from build123d import *

# Parameters (mm, degrees)
F0_R            = 75
F1_DEPTH        = 5
F2_W            = 78
F2_H            = 78
F2_W_2          = 76
F2_H_2          = 76
F2_W_3          = 56
F2_H_3          = 56
F2_W_4          = 54
F2_H_4          = 54
F3_DEPTH        = 1
F4_R            = 1
F5_DEPTH        = 5.001
F5_COPIES_COUNT = 3


# Not quite as in the source:
# - a pattern or mirror of a feature is missing from the dataset's text; its kind, count and spacing are read off the source's solid


with BuildPart() as f1:
    # F0 (on Top) → F1 (new body)
    with BuildSketch(Plane.XY):
        Circle(F0_R)
    extrude(amount=F1_DEPTH)

    # F2 (on face) → F3 (cut)
    with BuildSketch(Plane.XY.offset(5)):
        Rectangle(F2_W, F2_H)
        Rectangle(F2_W_2, F2_H_2, mode=Mode.SUBTRACT)
        Rectangle(F2_W_3, F2_H_3)
        Rectangle(F2_W_4, F2_H_4, mode=Mode.SUBTRACT)
    extrude(amount=-F3_DEPTH, mode=Mode.SUBTRACT)

    # F4 (on face) → F5 (cut, through all)
    with BuildSketch(Plane.XY.offset(5)):
        with Locations((0, 70)):
            Circle(F4_R)
        with Locations((3.663516937, 69.9040674328)):
            Circle(F4_R)
        with Locations((7.3169924287, 69.6165326758)):
            Circle(F4_R)
    f5 = extrude(amount=-F5_DEPTH, mode=Mode.SUBTRACT)

    # F5_copies: F5 ×3 about axis
    f5_copies_axis = Axis((0, 0, 0), (0, 0, 1))
    for i in range(1, F5_COPIES_COUNT):
        add(f5.rotate(f5_copies_axis, i * 360 / F5_COPIES_COUNT), mode=Mode.SUBTRACT)


solid = f1.part
Input: part model. Units: mm. Frame: model coordinates. Give positions to 0.01 mm unless a question says otherwise; leave off trailing zeros. Order: outer loops, then holes, each group sorted by start corner. A loop starts at its lowest first (then second) coordinate and runs counter-clockwise, first axis right, second up. Notation, with made-up numbers: M 2,-21.75 L 39,-21.75 A8 cw 39,-9.75 Z; hole C -22,85.25 d3. An arc over 180 degrees is marked long. Answer as a JSON object with one key per item and string values.
1. Cut plane B-B, the plane y = -18.5. Output: boundary loops of the cut face in (x, z).
Result sheet:
{"outline": "M -72.68,0 L 72.68,0 L 72.68,5 L 39,5 L 39,4 L 38,4 L 38,5 L 28,5 L 28,4 L 27,4 L 27,5 L -27,5 L -27,4 L -28,4 L -28,5 L -38,5 L -38,4 L -39,4 L -39,5 L -72.68,5 Z"}
2. Cut plane A-A, the plane z = 1. State how many separate pieces and enclosed holes the cut face has, and give its area (3 significant figures).
Result sheet:
{"separate pieces": "1", "enclosed holes": "9", "area": "17,600 mm²"}
3. Cut plane C-C, the plane x = -14. Output: boundary loops of the cut face in (y, z).
Result sheet:
{"outline": "M -73.68,0 L 73.68,0 L 73.68,5 L 39,5 L 39,4 L 38,4 L 38,5 L 28,5 L 28,4 L 27,4 L 27,5 L -27,5 L -27,4 L -28,4 L -28,5 L -38,5 L -38,4 L -39,4 L -39,5 L -73.68,5 Z"}
4. Cut plane D-D, the plane y = -45. Output: boundary loops of the cut face in (x, z).
Result sheet:
{"outline": "M -60,0 L 60,0 L 60,5 L -60,5 Z"}
5. Ray query, line 1 (Y direction, x = 0, z = 1.8); line 2 (X direction, y = -3, z = 4.75); line 3 (X direction, y = 29.5, z = 4.85). Return the intervals inside material, ascending. Write a range as [from, to].
Result sheet:
{"line 1": "[-75, 69], [71, 75]", "line 2": "[-74.94, -39], [-38, -28], [-27, 27], [28, 38], [39, 74.94]", "line 3": "[-68.95, -39], [-38, 38], [39, 68.95]"}
6. First-contact query: P1, Ø2, axis at y = 39.5, z = 2, coming from the +X side; P2, Ø1, axis at x = 6, z = 4.5, coming from the +Y side; P3, Ø0.5, axis at y = 4.5, z = 4.5, coming from the +X side; P4, Ø2.5, axis at x = -63.95, y = -28.47, coming from the +Z side. Flat tips, straight axial feed; report the tip coordinate or a pass-through.
Result sheet:
{"P1": "x = 64.36", "P2": "y = 74.8", "P3": "x = 74.88", "P4": "z = 5"}
